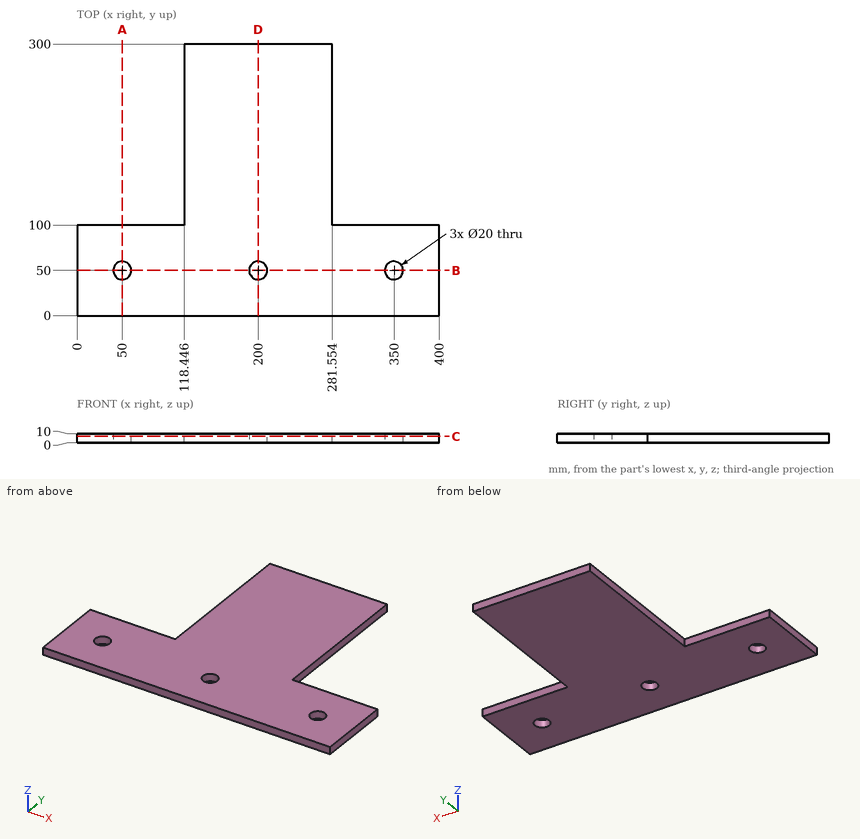
Geometry check sheet. Reference: drawing and pictorial views, mm from the part's lowest x, y, z. Coordinates: 2 decimals unless noted, no trailing zeros. Order: outer loops, then holes, each group sorted by start corner. A loop starts at its lowest first (then second) coordinate and runs counter-clockwise, first axis right, second up. Notation, with made-up numbers: M -31,47.5 L -2,47.5 A31 ccw -2,84.5 Z; hole C 1,69.5 d1. An arc over 180 degrees is marked long. Write each question's results on one line, items separated by ' | '. Start each with the question number.
1. Cross-section at C-C on z = 7. Record the cut outline in (x, y).
2. Cross-section at D-D on x = 200. Record the cut outline in (y, z), and give its area (3 significant figures).
3. Cross-section at A-A on x = 50. Record the cut outline in (y, z), and give its area (3 significant figures).
4. Material ranges on probe 1 along Y at (x, z) = (50, 5.75); probe 2 along Y at (x, z) = (200, 7.25); probe 3 along X at (y, z) = (251.5, 1.25), recorded low to high.
5. Cross-section at B-B on y = 50. Record the cut outline in (x, z).
6. Go/stop test with flat-tipped pins: P1, Ø3, axis at x = 81.5, z = 5, coming from the +Y side; P2, Ø3, axis at y = 155, z = 6, coming from the -X side; P3, Ø3, axis at y = 165, z = 5, coming from the +X side. Record where each tip stops, or that it passes through.
Checks:
1) outline: M 0,0 L 400,0 L 400,100 L 281.55,100 L 281.55,300 L 118.45,300 L 118.45,100 L 0,100 Z; hole C 50,50 d20; hole C 200,50 d20; hole C 350,50 d20
2) outline: M 0,0 L 40,0 L 40,10 L 0,10 Z; M 60,0 L 300,0 L 300,10 L 60,10 Z | area: 2,800 mm²
3) outline: M 0,0 L 40,0 L 40,10 L 0,10 Z; M 60,0 L 100,0 L 100,10 L 60,10 Z | area: 800 mm²
4) probe 1: y = 0 to 40, 60 to 100 | probe 2: y = 0 to 40, 60 to 300 | probe 3: x = 118.45 to 281.55
5) outline: M 0,0 L 40,0 L 40,10 L 0,10 Z; M 60,0 L 190,0 L 190,10 L 60,10 Z; M 210,0 L 340,0 L 340,10 L 210,10 Z; M 360,0 L 400,0 L 400,10 L 360,10 Z
6) P1: stops at y = 100 | P2: stops at x = 118.45 | P3: stops at x = 281.55
